```python
from build123d import *

# Parameters (mm, degrees)
SKETCH_1_W          = 68
SKETCH_1_H          = 68
SKETCH_1_R          = 17.5
EXTRUDE_1_DEPTH     = 4
SKETCH_2_W          = 12
SKETCH_2_H          = 4
SKETCH_2_W_2        = 4
SKETCH_2_H_2        = 12
EXTRUDE_2_DEPTH     = 4
SKETCH_3_R          = 1.5
CUT_EXTRUDE_1_DEPTH = 4
FILLET_1_R          = 3
SKETCH_4_R          = 2.1
CUT_EXTRUDE_2_DEPTH = 10


with BuildPart() as part:
    # 草图1 → 凸台-拉伸1 (new body)
    with BuildSketch(Plane(origin=(0, 0, 0), x_dir=(1, 0, 0), z_dir=(0, 1, 0))):
        Rectangle(SKETCH_1_W, SKETCH_1_H)
        with Locations(Location((0, 0, 0), (0, 0, 270))):
            Circle(SKETCH_1_R, mode=Mode.SUBTRACT)
    extrude(amount=EXTRUDE_1_DEPTH)

    # 草图2 → 凸台-拉伸2 (add)
    with BuildSketch(Plane(origin=(0, 4, 0), x_dir=(1, 0, 0), z_dir=(0, 1, 0))):
        with Locations((-15, 36)):
            Rectangle(SKETCH_2_W, SKETCH_2_H)
        with Locations((15, 36)):
            Rectangle(SKETCH_2_W, SKETCH_2_H)
        with Locations((36, 15)):
            Rectangle(SKETCH_2_W_2, SKETCH_2_H_2)
        with Locations((36, -15)):
            Rectangle(SKETCH_2_W_2, SKETCH_2_H_2)
        with Locations((15, -36)):
            Rectangle(SKETCH_2_W, SKETCH_2_H)
        with Locations((-15, -36)):
            Rectangle(SKETCH_2_W, SKETCH_2_H)
        with Locations((-36, -15)):
            Rectangle(SKETCH_2_W_2, SKETCH_2_H_2)
        with Locations((-36, 15)):
            Rectangle(SKETCH_2_W_2, SKETCH_2_H_2)
    extrude(amount=-EXTRUDE_2_DEPTH)

    # 草图3 → 切除-拉伸1 (cut)
    with BuildSketch(Plane(origin=(0, 4, 0), x_dir=(1, 0, 0), z_dir=(0, 1, 0))):
        with Locations((-22.5, 34)):
            Circle(SKETCH_3_R)
        with Locations((-7.5, 34)):
            Circle(SKETCH_3_R)
        with Locations((7.5, 34)):
            Circle(SKETCH_3_R)
        with Locations((22.5, 34)):
            Circle(SKETCH_3_R)
        with Locations((34, 22.5)):
            Circle(SKETCH_3_R)
        with Locations((34, 7.5)):
            Circle(SKETCH_3_R)
        with Locations((34, -7.5)):
            Circle(SKETCH_3_R)
        with Locations((34, -22.5)):
            Circle(SKETCH_3_R)
        with Locations((22.5, -34)):
            Circle(SKETCH_3_R)
        with Locations((7.5, -34)):
            Circle(SKETCH_3_R)
        with Locations((-7.5, -34)):
            Circle(SKETCH_3_R)
        with Locations((-22.5, -34)):
            Circle(SKETCH_3_R)
        with Locations((-34, -22.5)):
            Circle(SKETCH_3_R)
        with Locations((-34, -7.5)):
            Circle(SKETCH_3_R)
        with Locations((-34, 7.5)):
            Circle(SKETCH_3_R)
        with Locations((-34, 22.5)):
            Circle(SKETCH_3_R)
    extrude(amount=-CUT_EXTRUDE_1_DEPTH, mode=Mode.SUBTRACT)

    # 圆角1
    fillet_1_edges = [part.edges().sort_by_distance(p)[0] for p in [
        (34, 2, 34),
        (-34, 2, 34),
        (-34, 2, -34),
        (34, 2, -34),
    ]]
    fillet(fillet_1_edges, radius=FILLET_1_R)

    # 草图4 → 切除-拉伸2 (cut)
    with BuildSketch(Plane(origin=(0, 4, 0), x_dir=(1, 0, 0), z_dir=(0, 1, 0))):
        with Locations(Location((24, 0, 0), (0, 0, 270))):
            Circle(SKETCH_4_R)
        with Locations(Location((12, -20.784609691, 0), (0, 0, 270))):
            Circle(SKETCH_4_R)
        with Locations(Location((-12, -20.784609691, 0), (0, 0, 270))):
            Circle(SKETCH_4_R)
        with Locations(Location((-24, 0, 0), (0, 0, 270))):
            Circle(SKETCH_4_R)
        with Locations(Location((-12, 20.784609691, 0), (0, 0, 270))):
            Circle(SKETCH_4_R)
        with Locations(Location((12, 20.784609691, 0), (0, 0, 270))):
            Circle(SKETCH_4_R)
    extrude(amount=-CUT_EXTRUDE_2_DEPTH, mode=Mode.SUBTRACT)


solid = part.part
```
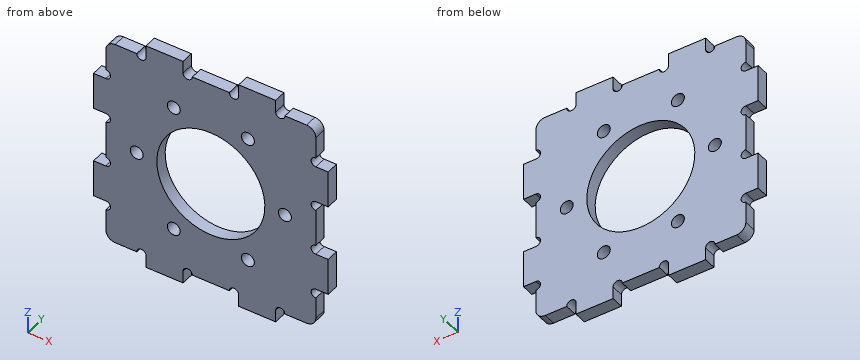
Part model, mm, in its own coordinate system. Give positions to 0.01 mm unless a question says otherwise; leave off trailing zeros. Write each loop counter-clockwise with the first axis right and the second up, starting at its lowest first coordinate (ties: lowest second). Pieces come first, ordered by that corner, then holes. Notation, with made-up numbers: (-13, -13.75) -> (25, -13.75) arc R10 cw to (25, -8.75) -> close; hole circle Ø2 at (23, 44.5). An arc over 180 degrees is marked (long way). Put each result on its own line as item: value. Start each with the question number.
Item 1: Cut at A-A (x = 0). List the corners of the cut face in (y, z), then the cut area to 3 significant figures.
Item 2: Wall check: L1, parallel to X at y = 0.9, z = 0; L2, parallel to X at y = 1.65, z = 20.5; L3, parallel to Z at x = 34.5, y = 3.75. Give the ranges that are in metal, low to high. Write a range as [from, to].
Item 3: Cut at C-C (y = 1.65). State how many separate pieces and enclosed holes the cut face has, then the cut area to 3 significant figures.
Item 4: Pin check, flat tips, straight feed: pin 1 Ø1.5 at (y, z) = (2.5, -2) entering from -X; pin 2 Ø6 at (x, z) = (10.5, 25.5) entering from -Y; pin 3 Ø2 at (y, z) = (2, 26.5) entering from +X; pin 4 Ø2 at (y, z) = (1.5, -37) entering from +X. Stop position of each tip, or through.
Item 5: Cut at B-B (z = 7.5). List the corners of the cut face in (x, y).
Item 6: Cut at D-D (x = -12). List the corners of the cut face in (y, z), then the cut area to 3 significant figures.
Answer list:
1. outline: (0, -34) -> (4, -34) -> (4, -17.5) -> (0, -17.5) -> close; (0, 17.5) -> (4, 17.5) -> (4, 34) -> (0, 34) -> close
1. area: 132 mm2
2. L1: x = [-34, -26.1], [-21.9, -17.5], [17.5, 21.9], [26.1, 34]
2. L2: x = [-38, -14.08], [-9.92, 9.92], [14.08, 38]
2. L3: z = [-21, -9], [9, 21]
3. separate pieces: 1
3. enclosed holes: 7
3. area: 3,900 mm2
4. pin 1: stops at x = -34
4. pin 2: stops at y = 0
4. pin 3: stops at x = 34
4. pin 4: stops at x = 21
5. outline: (-32.5, 0) -> (-15.81, 0) -> (-15.81, 4) -> (-32.5, 4) -> close; (15.81, 0) -> (32.5, 0) -> (32.5, 4) -> (15.81, 4) -> close
6. outline: (0, -38) -> (4, -38) -> (4, -22.88) -> (0, -22.88) -> close; (0, -18.68) -> (4, -18.68) -> (4, -12.74) -> (0, -12.74) -> close; (0, 12.74) -> (4, 12.74) -> (4, 18.68) -> (0, 18.68) -> close; (0, 22.88) -> (4, 22.88) -> (4, 38) -> (0, 38) -> close
6. area: 168 mm2
